For this review, use the dimensioned drawing (mm, ordinates from the lowest corner) and the shaded views. A direction names the side the tool comes from. Give positions to 0.01 mm unless a question says otherwise; leave off trailing zeros. Loops run counter-clockwise (first coordinate to the right, second up) from the corner with the lowest first, then second, coordinate; pieces in that order, holes last. Notation, with made-up numbers: (-39, 67.5) -> (-32, 67.5) arc R15 cw to (-32, 95.5) -> close; hole circle Ø11 at (2, 58). An arc over 180 degrees is marked (long way). Write each question's results on one line, items separated by ' | '. Start each with the question number.
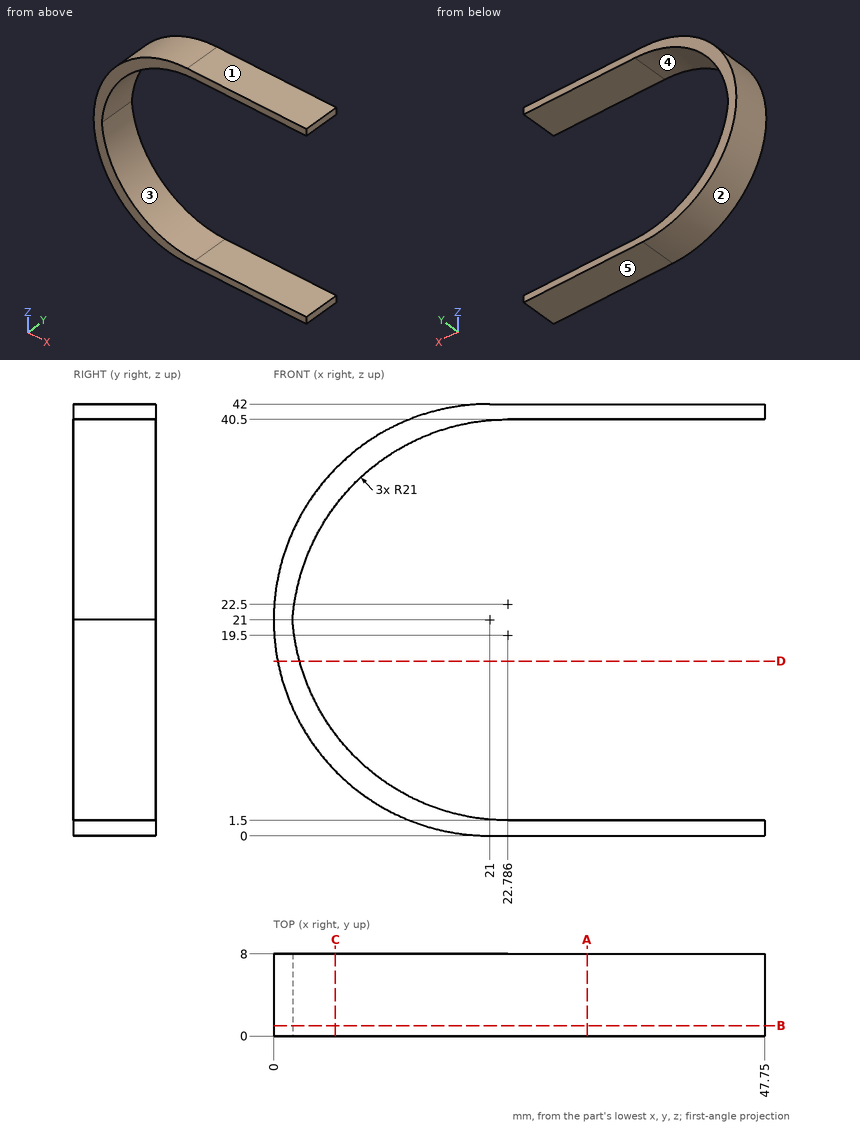
1. For pin 1 Ø4 at (y, z) = (1, 35) entering from +X; pin 2 Ø4 at (x, y) = (11, 3) entering from +Z; pin 3 Ø4 at (y, z) = (6.5, 16) entering from +X, all flat-tipped, find the tip position at first contact; note any pin that passes through.
2. Wall thickness on L1, parallel to Z at x = 30, y = 3.25; L2, parallel to Z at x = 13, y = 3.25; L3, parallel to X at y = 6.5, z = 30.5: over which ranges is each line inside the solid? List them lowest first.
3. Draft analysis for pull direction Z (two halves, no side actions). For the marked faces 1, 2 and 3, state which applies: released by +Z, released by -Z, zero draft, split by the parting line, or undercut.
4. We need section A-A (x = 30.5). Write out the cut boundary in (y, z), plus the area to 3 significant figures.
5. We need section B-B (y = 1). Write out the cut boundary in (x, z).
6. We need section C-C (x = 6). Write out the cut boundary in (y, z).
7. We need section D-D (z = 17). Write out the cut boundary in (x, y) (1 decimal).
8. Machinability: for the marked faces 4 and 5, which of the approach directions +Z, -Z, +X, -X, +Y, -Y give a long, thin tool a straight path to every point of the face, cutting with its end or side? Answer none if there is none.
Response:
1) pin 1: stops at x = 11.18 | pin 2: stops at z = 40.42 | pin 3: stops at x = 3.58
2) L1: z = 0 to 1.5, 40.5 to 42 | L2: z = 1.58 to 3.92, 38.08 to 40.42 | L3: x = 2.27 to 4.9
3) face 1: released by +Z | face 2: split by the parting line | face 3: undercut
4) outline: (0, 0) -> (8, 0) -> (8, 1.5) -> (0, 1.5) -> close; (0, 40.5) -> (8, 40.5) -> (8, 42) -> (0, 42) -> close | area: 24.0 mm2
5) outline: (1.84, 21) arc R21 cw to (22.79, 40.5) -> (47.75, 40.5) -> (47.75, 42) -> (21, 42) arc R21 ccw to (21, 0) -> (47.75, 0) -> (47.75, 1.5) -> (22.79, 1.5) arc R21 cw to start
6) outline: (0, 6.3) -> (8, 6.3) -> (8, 9.88) -> (0, 9.88) -> close; (0, 32.12) -> (8, 32.12) -> (8, 35.7) -> (0, 35.7) -> close
7) outline: (0.4, 0) -> (2.5, 0) -> (2.5, 8) -> (0.4, 8) -> close
8) face 4: +X, +Y, -Y | face 5: -Z, +X, -X, +Y, -Y
